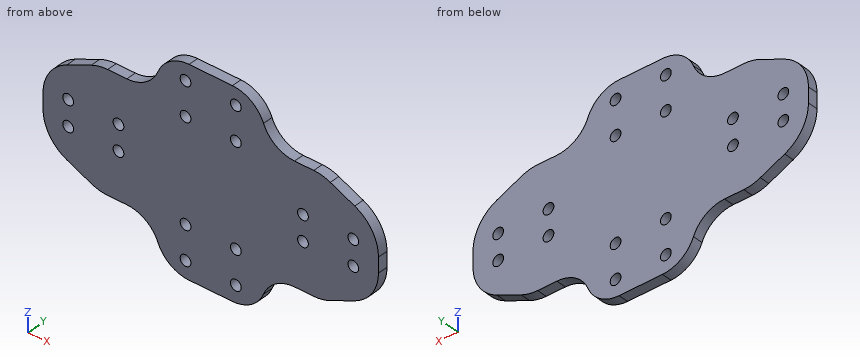
from build123d import *

# Parameters (mm, degrees)
SKETCH_2_W          = 30
SKETCH_2_H          = 60
SKETCH_2_R          = 1.6
EXTRUDE_1_DEPTH     = 3
SKETCH_3_W          = 100
SKETCH_3_H          = 35
SKETCH_3_W_2        = 28.612944684
SKETCH_3_H_2        = 33.572555392
EXTRUDE_2_DEPTH     = 3
SKETCH_4_R          = 1.6
CUT_EXTRUDE_1_DEPTH = 59.386642308
SKETCH_6_OUTSIDE_W  = 125.332
SKETCH_6_OUTSIDE_H  = 85.332
CUT_EXTRUDE_2_DEPTH = 59.386642308
FILLET_3_R          = 10
FILLET_4_R          = 10
FILLET_5_R          = 12
FILLET_6_R          = 12


with BuildPart() as part:
    # 草图2 → 凸台-拉伸1 (new body)
    with BuildSketch(Plane(origin=(0, 0, 0), x_dir=(1, 0, 0), z_dir=(0, 1, 0))):
        Rectangle(SKETCH_2_W, SKETCH_2_H)
        with Locations(Location((-7.5, -15, 0), (0, 0, 270))):
            Circle(SKETCH_2_R, mode=Mode.SUBTRACT)
        with Locations(Location((7.5, -15, 0), (0, 0, 270))):
            Circle(SKETCH_2_R, mode=Mode.SUBTRACT)
        with Locations(Location((7.5, 15, 0), (0, 0, 270))):
            Circle(SKETCH_2_R, mode=Mode.SUBTRACT)
        with Locations(Location((7.5, 25, 0), (0, 0, 270))):
            Circle(SKETCH_2_R, mode=Mode.SUBTRACT)
        with Locations(Location((-7.5, 15, 0), (0, 0, 270))):
            Circle(SKETCH_2_R, mode=Mode.SUBTRACT)
        with Locations(Location((-7.5, 25, 0), (0, 0, 270))):
            Circle(SKETCH_2_R, mode=Mode.SUBTRACT)
        with Locations(Location((7.5, -25, 0), (0, 0, 270))):
            Circle(SKETCH_2_R, mode=Mode.SUBTRACT)
        with Locations(Location((-7.5, -25, 0), (0, 0, 270))):
            Circle(SKETCH_2_R, mode=Mode.SUBTRACT)
    extrude(amount=EXTRUDE_1_DEPTH)

    # 草图3 → 凸台-拉伸2 (add)
    with BuildSketch(Plane.XZ):
        Rectangle(SKETCH_3_W, SKETCH_3_H)
        Rectangle(SKETCH_3_W_2, SKETCH_3_H_2, mode=Mode.SUBTRACT)
    extrude(amount=-EXTRUDE_2_DEPTH)

    # 草图4 → 切除-拉伸1 (cut, through all)
    with BuildSketch(Plane.XZ):
        with Locations(Location((-42.5, 3.75, 0), (0, 0, 270))):
            Circle(SKETCH_4_R)
        with Locations(Location((-42.5, -3.75, 0), (0, 0, 90))):
            Circle(SKETCH_4_R)
        with Locations(Location((-27.5, -3.75, 0), (0, 0, 270))):
            Circle(SKETCH_4_R)
        with Locations(Location((-27.5, 3.75, 0), (0, 0, 90))):
            Circle(SKETCH_4_R)
        with Locations(Location((42.5, 3.75, 0), (0, 0, 90))):
            Circle(SKETCH_4_R)
        with Locations(Location((42.5, -3.75, 0), (0, 0, 270))):
            Circle(SKETCH_4_R)
        with Locations(Location((27.5, -3.75, 0), (0, 0, 90))):
            Circle(SKETCH_4_R)
        with Locations(Location((27.5, 3.75, 0), (0, 0, 270))):
            Circle(SKETCH_4_R)
    extrude(amount=-CUT_EXTRUDE_1_DEPTH, mode=Mode.SUBTRACT)

    # 草图6 outside → 切除-拉伸2 (cut, through all)
    with BuildSketch(Plane(origin=(0, 3, 0), x_dir=(1, 0, 0), z_dir=(0, 1, 0))):
        Rectangle(SKETCH_6_OUTSIDE_W, SKETCH_6_OUTSIDE_H)
        Polygon((-15, 30), (-23.291561976, 17.5), (-33.291561976, 17.5), (-50, 10), (-50, -10), (-33.291561976, -17.5), (-23.291561976, -17.5), (-15, -30), (15, -30), (23.291561976, -17.5), (33.291561976, -17.5), (50, -10), (50, 10), (33.291561976, 17.5), (23.291561976, 17.5), (15, 30), align=None, mode=Mode.SUBTRACT)
    extrude(amount=-CUT_EXTRUDE_2_DEPTH, mode=Mode.SUBTRACT)

    # 圆角3
    fillet_3_edges = [part.edges().sort_by_distance(p)[0] for p in [
        (15, 1.5, -17.5),
        (15, 1.5, 17.5),
        (-15, 1.5, -17.5),
        (-15, 1.5, 17.5),
    ]]
    fillet(fillet_3_edges, radius=FILLET_3_R)

    # 圆角4
    fillet_4_edges = [part.edges().sort_by_distance(p)[0] for p in [
        (-15, 1.5, 30),
        (15, 1.5, 30),
        (15, 1.5, -30),
        (-15, 1.5, -30),
    ]]
    fillet(fillet_4_edges, radius=FILLET_4_R)

    # 圆角5
    fillet_5_edges = [part.edges().sort_by_distance(p)[0] for p in [
        (50, 1.5, -10),
        (50, 1.5, 10),
        (-50, 1.5, 10),
        (-50, 1.5, -10),
    ]]
    fillet(fillet_5_edges, radius=FILLET_5_R)

    # 圆角6
    fillet_6_edges = [part.edges().sort_by_distance(p)[0] for p in [
        (33.291561976, 1.5, -17.5),
        (33.291561976, 1.5, 17.5),
        (-33.291561976, 1.5, 17.5),
        (-33.291561976, 1.5, -17.5),
    ]]
    fillet(fillet_6_edges, radius=FILLET_6_R)


solid = part.part
Can you work these out from the model? Positions are in its coordinate system, mm. Give positions to 0.01 mm unless a question says otherwise; leave off trailing zeros. Write each loop counter-clockwise with the first axis right and the second up, starting at its lowest first coordinate (ties: lowest second). Pieces come first, ordered by that corner, then holes. Notation, with made-up numbers: (75.25, 40.25) -> (125.25, 40.25) arc R30 cw to (125.25, 73.25) -> close; hole circle Ø5 at (43, 0). An arc over 180 degrees is marked (long way). Answer as a JSON object with one key per item and string values. Group by question number.
Item 1: Please list where these lines run through material, in increasing order: line 1 (X direction, y = 0.6, z = 14.5); line 2 (X direction, y = 1.6, z = 3.75); line 3 (X direction, y = 1.9, z = -26). Write a range as [from, to].
Item 2: Suppose I cut it at A-A (x = -27.5). Please give me the cut outline in (y, z).
Item 3: Suppose I cut it at B-B (z = 3.75). Please give me the cut outline in (x, y), plus the area to 3 significant figures.
Item 4: Suppose I cut it at D-D (z = 15). Please give me the cut outline in (x, y), plus the area to 3 significant figures.
Item 5: I'm going to push flat-ended pins straight in: P1, Ø1.5, axis at x = -27, y = 1, coming from the -Z side; P2, Ø1.9, axis at x = 7.5, z = -15, coming from the -Y side. Where does each tip first touch, or does it pass through?
Item 6: Suppose I cut it at C-C (y = 1.4). State how many separate pieces and enclosed holes the cut face has, plus the area to 3 significant figures.
Findings:
{
 "1": {"line 1": "x = [-39.97, -9.02], [-5.98, 5.98], [9.02, 39.97]", "line 2": "x = [-49.9, -44.1], [-40.9, -29.1], [-25.9, 25.9], [29.1, 40.9], [44.1, 49.9]", "line 3": "x = [-14.46, -8.75], [-6.25, 6.25], [8.75, 14.46]"},
 "2": {"outline": "(0, -17.5) -> (3, -17.5) -> (3, -5.35) -> (0, -5.35) -> close; (0, -2.15) -> (3, -2.15) -> (3, 2.15) -> (0, 2.15) -> close; (0, 5.35) -> (3, 5.35) -> (3, 17.5) -> (0, 17.5) -> close"},
 "3": {"outline": "(-49.9, 0) -> (-44.1, 0) -> (-44.1, 3) -> (-49.9, 3) -> close; (-40.9, 0) -> (-29.1, 0) -> (-29.1, 3) -> (-40.9, 3) -> close; (-25.9, 0) -> (25.9, 0) -> (25.9, 3) -> (-25.9, 3) -> close; (29.1, 0) -> (40.9, 0) -> (40.9, 3) -> (29.1, 3) -> close; (44.1, 0) -> (49.9, 0) -> (49.9, 3) -> (44.1, 3) -> close", "area": "261 mm²"},
 "4": {"outline": "(-38.86, 0) -> (-9.1, 0) -> (-9.1, 3) -> (-38.86, 3) -> close; (-5.9, 0) -> (5.9, 0) -> (5.9, 3) -> (-5.9, 3) -> close; (9.1, 0) -> (38.86, 0) -> (38.86, 3) -> (9.1, 3) -> close", "area": "214 mm²"},
 "5": {"P1": "stops at z = -17.5", "P2": "passes through"},
 "6": {"separate pieces": "1", "enclosed holes": "16", "area": "3,860 mm²"}
}
